from build123d import *

# Parameters (mm, degrees)
SKETCH1_W           = 76.2
SKETCH1_H           = 38.1
BOSS_EXTRUDE1_DEPTH = 6.35
SKETCH2_W           = 76.2
SKETCH2_H           = 76.2
SKETCH2_R           = 4.1656
BOSS_EXTRUDE2_DEPTH = 6.35
SKETCH3_W           = 64.7
SKETCH3_H           = 57.7
SKETCH3_W_2         = 52
SKETCH3_H_2         = 45
BOSS_EXTRUDE3_DEPTH = 150
SKETCH4_W           = 64.7
SKETCH4_H           = 57.7
BOSS_EXTRUDE4_DEPTH = 6.35


with BuildPart() as part:
    # Sketch1 → Boss-Extrude1 (new body)
    with BuildSketch(Plane(origin=(0, 0, 0), x_dir=(1, 0, 0), z_dir=(0, 1, 0))):
        Rectangle(SKETCH1_W, SKETCH1_H)
    extrude(amount=BOSS_EXTRUDE1_DEPTH)

    # Sketch2 → Boss-Extrude2 (add)
    with BuildSketch(Plane(origin=(0, 0, -19.05), x_dir=(-1, 0, 0), z_dir=(0, 0, -1))):
        with Locations((0, -31.75)):
            Rectangle(SKETCH2_W, SKETCH2_H)
        with Locations((-19.05, -12.7)):
            Circle(SKETCH2_R, mode=Mode.SUBTRACT)
        with Locations((19.05, -12.7)):
            Circle(SKETCH2_R, mode=Mode.SUBTRACT)
        with Locations((19.05, -50.8)):
            Circle(SKETCH2_R, mode=Mode.SUBTRACT)
        with Locations((-19.05, -50.8)):
            Circle(SKETCH2_R, mode=Mode.SUBTRACT)
    extrude(amount=BOSS_EXTRUDE2_DEPTH)

    # Sketch3 → Boss-Extrude3 (add)
    with BuildSketch(Plane(origin=(0, 6.35, 0), x_dir=(1, 0, 0), z_dir=(0, 1, 0))):
        with Locations((70.45, 9.8)):
            Rectangle(SKETCH3_W, SKETCH3_H)
        with Locations((70.45, 9.8)):
            Rectangle(SKETCH3_W_2, SKETCH3_H_2, mode=Mode.SUBTRACT)
    extrude(amount=-BOSS_EXTRUDE3_DEPTH)

    # Sketch4 → Boss-Extrude4 (add)
    with BuildSketch(Plane.XZ.offset(143.65)):
        with Locations((70.45, -9.8)):
            Rectangle(SKETCH4_W, SKETCH4_H)
    extrude(amount=BOSS_EXTRUDE4_DEPTH)


solid = part.part
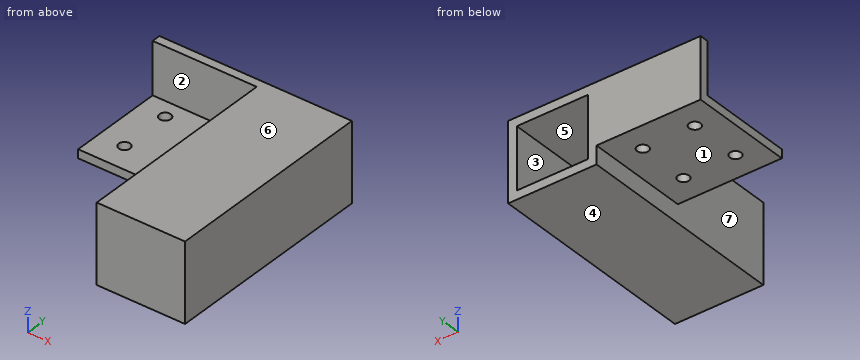
Part model, mm, in its own coordinate system. Face numbers are marked on the shaded views. A direction names the side the tool comes from. Coordinates: 2 decimals unless noted, no trailing zeros. Order: outer loops, then holes, each group sorted by start corner. A loop starts at its lowest first (then second) coordinate and runs counter-clockwise, first axis right, second up.
(1) Probe L1, parallel to Y at x = 19.05, z = -22.75; L2, parallel to X at y = -41, z = -12; L3, parallel to Z at x = 84, y = -0.5. List the from-to ranges inside material, lowest first.
Check sheet entries:
L1: y = -69.85 to -54.97, -46.63 to -16.87, -8.53 to 6.35
L2: x = 38.1 to 44.45, 96.45 to 102.8
L3: z = -38.65 to -32.3, 12.7 to 19.05
(2) Slice it at A-A, the plane y = -12.7. Write the cut outline in (x, z).
Check sheet entries:
outline: (-38.1, -25.4) - (-23.22, -25.4) - (-23.22, -19.05) - (-38.1, -19.05) - close; (-14.88, -25.4) - (14.88, -25.4) - (14.88, -19.05) - (-14.88, -19.05) - close; (23.22, -25.4) - (38.1, -25.4) - (38.1, -38.65) - (102.8, -38.65) - (102.8, 19.05) - (38.1, 19.05) - (38.1, -19.05) - (23.22, -19.05) - close; hole (44.45, -32.3) - (96.45, -32.3) - (96.45, 12.7) - (44.45, 12.7) - close
(3) Slice it at C-C, the plane y = -82.5. Write the cut outline in (x, z).
Check sheet entries:
outline: (38.1, -38.65) - (102.8, -38.65) - (102.8, 19.05) - (38.1, 19.05) - close; hole (44.45, -32.3) - (96.45, -32.3) - (96.45, 12.7) - (44.45, 12.7) - close
(4) Slice it at D-D, the plane z = 6. Write the cut outline in (x, y).
Check sheet entries:
outline: (-38.1, 0) - (38.1, 0) - (38.1, -150) - (102.8, -150) - (102.8, 6.35) - (96.45, 6.35) - (96.45, -143.65) - (44.45, -143.65) - (44.45, 6.35) - (-38.1, 6.35) - close
(5) Pull direction Z, two halves, no side cores. Call the marked faces 4, 5, 6 and 7: pulls with the +Z half, pulls with the -Z half, needs draft (parallel to the pull), parting line crosses it, or undercut.
Check sheet entries:
face 4: pulls with the -Z half
face 5: undercut
face 6: pulls with the +Z half
face 7: needs draft
(6) Pin check, flat tips, straight feed: pin 1 Ø4 at (x, z) = (18.5, -18) entering from -Y; pin 2 Ø5 at (x, y) = (12, -53) entering from +Z; pin 3 Ø7.5 at (x, y) = (19.05, -12.7) entering from +Z; pin 4 Ø4 at (x, z) = (51.5, 7) entering from +Y. Stop position of each tip, or through.
Check sheet entries:
pin 1: stops at y = -69.85
pin 2: stops at z = -19.05
pin 3: passes through
pin 4: stops at y = -143.65
(7) Tool access for the marked faces 1, 2 and 3: list every direction of +Z, -Z, +X, -X, +Y, -Y with a clear straight run to the whole face (end or side of a thin tool).
Check sheet entries:
face 1: -Z, -X, +Y, -Y
face 2: +Z, -X, -Y
face 3: +Y
(8) Slice it at B-B, the plane x = -19.05. Write the cut outline in (y, z).
Check sheet entries:
outline: (-69.85, -25.4) - (-54.97, -25.4) - (-54.97, -19.05) - (-69.85, -19.05) - close; (-46.63, -25.4) - (-16.87, -25.4) - (-16.87, -19.05) - (-46.63, -19.05) - close; (-8.53, -25.4) - (6.35, -25.4) - (6.35, 19.05) - (0, 19.05) - (0, -19.05) - (-8.53, -19.05) - close
